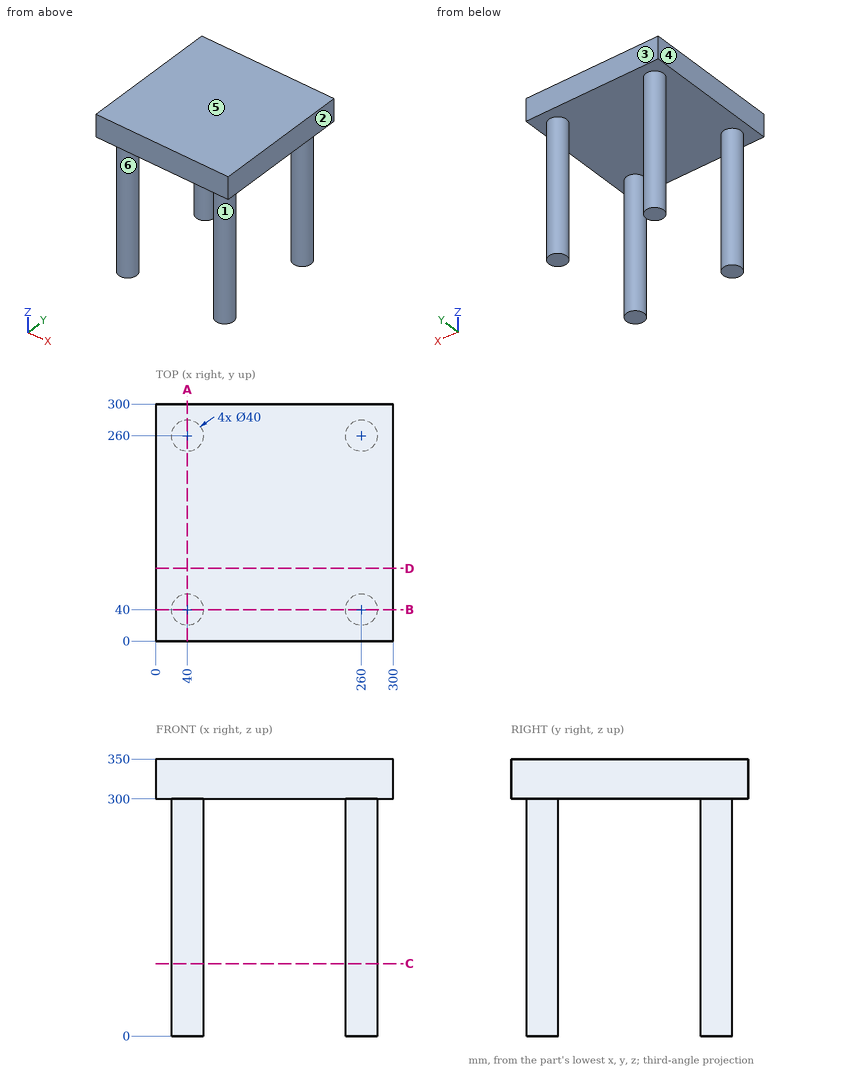
Print and shaded views of the part. All mm, measured from the part's lowest x, y and z. A direction names the side the tool comes from. Coordinates: 2 decimals unless noted, no trailing zeros. Loops run counter-clockwise (first coordinate to the right, second up) from the corner with the lowest first, then second, coordinate; pieces in that order, holes last. Notation, with made-up numbers: (-22.75, 73.5) - (1.25, 73.5) arc R32 ccw to (1.25, 101.5) - close; hole circle Ø11 at (73.5, 87.25). An arc over 180 degrees is marked (long way). Use one line per item in the form item = value. Start each with the question number.
1) Drill centre lines: L1, parallel to Z at x = 34, y = 101.5; L2, parallel to Y at x = 278, z = 186; L3, parallel to Y at x = 262.5, z = 262. Where is each one in solid material? Low to high. Write a range as from..to.
2) Band-saw the part on C-C (z = 91.5). Give the cut face in (x, y), and give its area (3 significant figures).
3) Tool access for the marked faces 5 and 6: list every direction of +Z, -Z, +X, -X, +Y, -Y with a clear straight run to the whole face (end or side of a thin tool).
4) Flat gauge pins, fed straight in: pin 1 (2 mm diameter, centred on x = 55.5, z = 215, fed in from +Y) (3 decimals); pin 2 (1 mm diameter, centred on x = 145, y = 101.5, fed in from -Z). Where does each tip first touch, or does it go through?
5) Band-saw the part on D-D (y = 92). Give the cut face in (x, z), and give its area (3 significant figures).
6) Band-saw the part on A-A (x = 40). Give the cut face in (y, z), and give its area (3 significant figures).
7) Two-plate mould, pull along X, no slides. Class the marked faces 1, 2, 3 and 4: +X half, -X half, draft (parallel to the pull), parting line (faces both ways), or undercut.
Check values:
q1.L1 = 300..350
q1.L2 = 31.28..48.72, 251.28..268.72
q1.L3 = 20.16..59.84, 240.16..279.84
q2.outline = circle Ø40 at (40, 40); circle Ø40 at (40, 260); circle Ø40 at (260, 40); circle Ø40 at (260, 260)
q2.area = 5,030 mm2
q3.face_5 = +Z, +X, -X, +Y, -Y
q3.face_6 = -Z
q4.pin_1 = 273.775
q4.pin_2 = 300
q5.outline = (0, 300) - (300, 300) - (300, 350) - (0, 350) - close
q5.area = 15,000 mm2
q6.outline = (0, 300) - (20, 300) - (20, 0) - (60, 0) - (60, 300) - (240, 300) - (240, 0) - (280, 0) - (280, 300) - (300, 300) - (300, 350) - (0, 350) - close
q6.area = 39,000 mm2
q7.face_1 = undercut
q7.face_2 = +X half
q7.face_3 = draft
q7.face_4 = -X half
